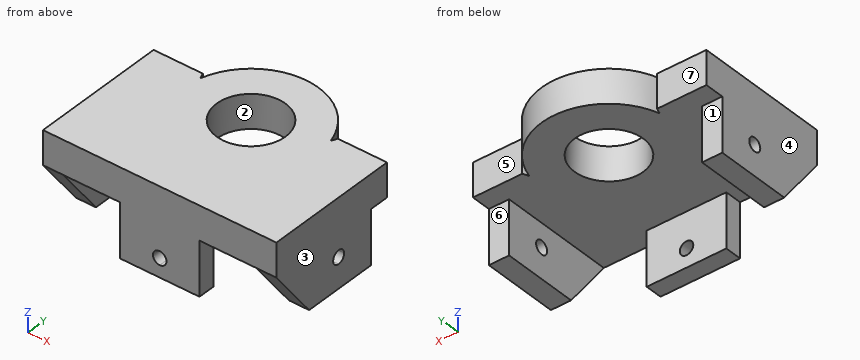
```python
from build123d import *

# Parameters (mm, degrees)
F0_R     = 12.7
F0_R_2   = 6.477
F1_DEPTH = 6.35
F3_DEPTH = 6.35
F5_DEPTH = 3.81
F7_DEPTH = 10.16
F9_DEPTH = 25.4


# Not quite as in the source:
# - a pattern or mirror of a feature is missing from the dataset's text; its kind, count and spacing are read off the source's solid


with BuildPart() as f1:
    # F0 (on Top) → F1 (new body)
    with BuildSketch(Plane.XY):
        Circle(F0_R)
        Circle(F0_R_2, mode=Mode.SUBTRACT)
    extrude(amount=F1_DEPTH)

    # F2 (on face) → F3 (join)
    with BuildSketch(Plane.XY.offset(6.35)):
        Polygon((-21.971, -21.0888834), (0, -21.0888834), (21.971, -21.0888834), (21.971, -17.9138834), (21.971, 4.445), (12.7, 4.445), (6.7730685696, -9.7721947122), (-6.9460314699, -9.7721947122), (-12.7, 4.445), (-21.971, 4.445), (-21.971, -17.907), align=None)
    extrude(amount=-F3_DEPTH)

    # F4 (on face) → F5 (join)
    with BuildSketch(Plane.YZ.offset(21.971)):
        Polygon((0.7805166, 6.35), (-21.0888834, 6.35), (-21.0888834, 0), (-13.5309724137, -10.16), (-6.7194938, -10.16), (0.7805166, -10.16), align=None)
        with BuildLine():
            ThreePointArc((-5.4494938, -4.445), (-5.8214681879, -5.3430256121), (-6.7194938, -5.715))
            ThreePointArc((-6.7194938, -5.715), (-7.6175194121, -3.5469743879), (-5.4494938, -4.445))
        make_face(mode=Mode.SUBTRACT)
    f5 = extrude(amount=-F5_DEPTH)

    # F5_copies: F5 across plane
    add(f5.mirror(Plane(origin=(0, 0, 0), x_dir=(0, 0, -1), z_dir=(-1, 0, 0))))

    # F6 (on face) → F7 (join)
    with BuildSketch(Plane(origin=(0, 0, 0), x_dir=(1, 0, 0), z_dir=(0, 0, -1))):
        Polygon((7.493, 21.0888834), (0, 21.0888834), (-7.493, 21.0888834), (-7.493, 17.9138834), (7.493, 17.9138834), align=None)
    extrude(amount=F7_DEPTH)

    # F8 (on face) → F9 (cut)
    with BuildSketch(Plane(origin=(0, -17.9138834, 0), x_dir=(-1, 0, 0), z_dir=(0, 1, 0))):
        with BuildLine():
            ThreePointArc((0, -7.912179098), (0.8980256121, -7.5402047101), (1.27, -6.642179098))
            ThreePointArc((1.27, -6.642179098), (-0.8980256121, -5.7441534859), (0, -7.912179098))
        make_face()
    extrude(amount=-F9_DEPTH, mode=Mode.SUBTRACT)


solid = f1.part
```
Geometry check sheet. Reference: the model listing, model coordinates, mm. Face numbers are marked on the shaded views. A direction names the side the tool comes from. Give positions to 0.01 mm unless a question says otherwise; leave off trailing zeros. Order: outer loops, then holes, each group sorted by start corner. A loop starts at its lowest first (then second) coordinate and runs counter-clockwise, first axis right, second up. Notation, with made-up numbers: (71.5, 50) - (104.5, 50) arc R12 ccw to (104.5, 65) - close; hole circle Ø11 at (-8.5, -17). An arc over 180 degrees is marked (long way). Answer in a Markdown table with one row per item. Add a question column.
Q1. Material ranges on probe 1 along X at (y, z) = (-14.5, -4.5); probe 2 along Z at (x, y) = (-16, -8.5); probe 3 along Y at (x, z) = (-4, 0.75), recorded low to high. Write a range as from..to.
Q2. Mould release check, pull along X, two halves, no side actions. Record for the marked faces 1, 2, 3 and 4: pulls with the +X half, pulls with the -X half, needs draft (parallel to the pull), parting line crosses it, or undercut.
Q3. Tool access check on the marked faces 5, 6 and 7. Record the directions out of +Z, -Z, +X, -X, +Y, -Y that give a thin tool (end or side, any length) a straight path to the whole face; none if there is none.
Q4. Cross-section at D-D, the plane z = -1.5. Enter the section's corners in (x, y).
Q5. Cross-section at A-A, the plane z = 5.5. Enter the section's corners in (x, y) (3 decimals).
Q6. Cross-section at C-C, the plane y = -11. Enter the section's corners in (x, z).
Q7. Gauge pin test, flat ends, axial feed: pin 1 (5 mm diameter, centred on x = 16, z = 4, fed in from +Y) (3 decimals); pin 2 (1.6 mm diameter, centred on y = -20, z = -6, fed in from +X); pin 3 (1.1 mm diameter, centred on x = 20.5, z = -3, fed in from +Y). Record the tip position at first contact, or that the pin passes through.
Q8. Cross-section at B-B, the plane y = 0. Enter the section's corners in (x, z).
Check values:
| question | item | result |
|---|---|---|
| 1 | probe 1 | x = -21.97..-18.16, 18.16..21.97 |
| 1 | probe 2 | z = 0..6.35 |
| 1 | probe 3 | y = -21.09..-5.09, 5.09..12.05 |
| 2 | face 1 | needs draft |
| 2 | face 2 | undercut |
| 2 | face 3 | pulls with the +X half |
| 2 | face 4 | pulls with the -X half |
| 3 | face 5 | +Z, -Z, +X, +Y |
| 3 | face 6 | -Z, +X, -X, +Y |
| 3 | face 7 | +Z, -Z, -X, +Y |
| 4 | outline | (-21.97, -19.97) - (-18.16, -19.97) - (-18.16, 0.78) - (-21.97, 0.78) - close; (-7.49, -21.09) - (7.49, -21.09) - (7.49, -17.91) - (-7.49, -17.91) - close; (18.16, -19.97) - (21.97, -19.97) - (21.97, 0.78) - (18.16, 0.78) - close |
| 5 | outline | (-21.971, -21.089) - (21.971, -21.089) - (21.971, 4.445) - (12.7, 4.445) - (12.248, 3.36) arc R12.7 ccw to (-12.253, 3.34) - (-12.7, 4.445) - (-21.971, 4.445) - close; hole circle Ø12.954 at (0, 0) |
| 6 | outline | (-21.97, -10.16) - (-18.16, -10.16) - (-18.16, 0) - (18.16, 0) - (18.16, -10.16) - (21.97, -10.16) - (21.97, 6.35) - (-21.97, 6.35) - close |
| 7 | pin 1 | stops at y = 4.445 |
| 7 | pin 2 | stops at x = 7.49 |
| 7 | pin 3 | stops at y = 0.78 |
| 8 | outline | (-21.97, -10.16) - (-18.16, -10.16) - (-18.16, 0) - (-6.48, 0) - (-6.48, 6.35) - (-21.97, 6.35) - close; (6.48, 0) - (18.16, 0) - (18.16, -10.16) - (21.97, -10.16) - (21.97, 6.35) - (6.48, 6.35) - close |
